Print and shaded views of the part. All mm, measured from the part's lowest x, y and z. A direction names the side the tool comes from. Coordinates: 2 decimals unless noted, no trailing zeros. Order: outer loops, then holes, each group sorted by start corner. A loop starts at its lowest first (then second) coordinate and runs counter-clockwise, first axis right, second up. Notation, with made-up numbers: M 12,11 L 35,11 A29 ccw 35,45 Z; hole C 11.25,0.5 d8. An arc over 180 degrees is marked long. Return JSON: item names as keys, results as strings.
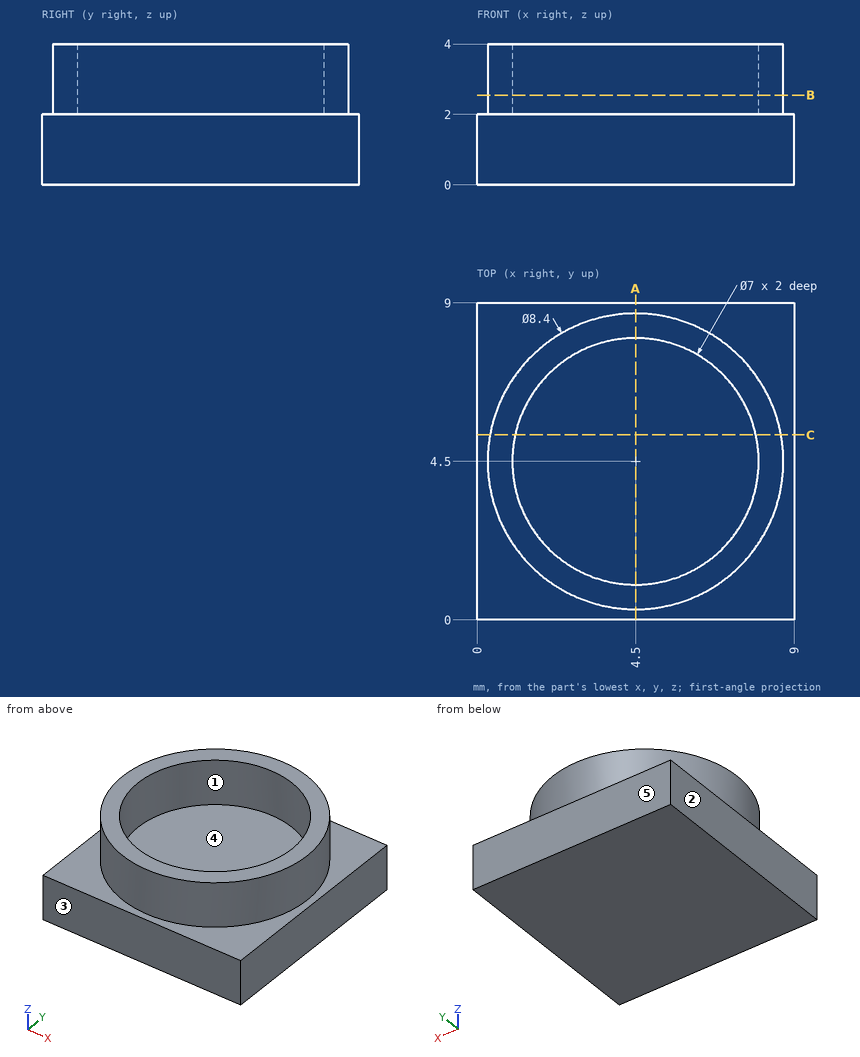
Item 1: Wall check: line 1 (Y direction, x = 4.5, z = 2.65); line 2 (Z direction, x = 0.75, y = 1.75); line 3 (X direction, y = 7.5, z = 2.9). Give the ranges that are in metal, low to high.
Check result:
{"line 1": "y = 0.3 to 1, 8 to 8.7", "line 2": "z = 0 to 2", "line 3": "x = 1.56 to 2.7, 6.3 to 7.44"}
Item 2: 3-axis set-ups, long thin cutter, end or side, ignore diameter. For the marked faces 4 and 5: which of +Z, -Z, +X, -X, +Y, -Y reach the whole face in a straight line?
Check result:
{"face 4": "+Z", "face 5": "+Z, -Z, +X, -X, +Y"}
Item 3: Drop flat-ended pins along their axis: pin 1 Ø2.5 at (x, y) = (4.5, 4) entering from +Z; pin 2 Ø1 at (y, z) = (3.5, 3.5) entering from -X; pin 3 Ø1.5 at (y, z) = (4.5, 3) entering from +X. Give the stop position or say it passes through.
Check result:
{"pin 1": "stops at z = 2", "pin 2": "stops at x = 0.33", "pin 3": "stops at x = 8.7"}
Item 4: Pull direction Y, two halves, no side cores. Call the marked faces 1, 2 and 3: +Y half, -Y half, draft (parallel to the pull), parting line (faces both ways), or undercut.
Check result:
{"face 1": "undercut", "face 2": "draft", "face 3": "-Y half"}
Item 5: Saw through at B-B (z = 2.55). Write the cut outline in (x, y).
Check result:
{"outline": "C 4.5,4.5 d8.4; hole C 4.5,4.5 d7"}
Item 6: Saw through at C-C (y = 5.25). Write the cut outline in (x, z).
Check result:
{"outline": "M 0,0 L 9,0 L 9,2 L 8.63,2 L 8.63,4 L 7.92,4 L 7.92,2 L 1.08,2 L 1.08,4 L 0.37,4 L 0.37,2 L 0,2 Z"}
Item 7: Saw through at A-A (x = 4.5). Write the cut outline in (y, z).
Check result:
{"outline": "M 0,0 L 9,0 L 9,2 L 8.7,2 L 8.7,4 L 8,4 L 8,2 L 1,2 L 1,4 L 0.3,4 L 0.3,2 L 0,2 Z"}
